from build123d import *

# Parameters (mm, degrees)
F0_W        = 12.9999973349
F0_H        = 13
F0_W_2      = 10
F0_H_2      = 10
F1_DEPTH    = 95
F2_T1_DEPTH = 38
F3_R        = 4
F4_DEPTH    = 2
F5_R        = 7
F5_R_2      = 4
F6_DEPTH    = 2


# Not quite as in the source:
# - a fillet or chamfer that OpenCascade refuses, or shapes differently, is made with other operations: its cross-section is extruded or revolved along the edge and cut away or added


with BuildPart() as f1:
    # F0 (on Right) → F1 (new body)
    with BuildSketch(Plane.YZ):
        with Locations((-12.2499999048, 6.5)):
            Rectangle(F0_W, F0_H)
        with Locations((-12.2499999048, 6.5)):
            Rectangle(F0_W_2, F0_H_2, mode=Mode.SUBTRACT)
    extrude(amount=F1_DEPTH)

    # F2: fillet of radius 5 on 2 edges, made by hand

    # F2_s2 → F2_t1 (cut)
    with BuildSketch(Plane.XY.offset(-12.5)):
        with BuildLine():
            ThreePointArc((90, -5.7500012374), (93.5355339059, -7.2144673315), (95, -10.7500012374))
            Line((95, -10.7500012374), (95, -5.7500012374))
            Line((95, -5.7500012374), (90, -5.7500012374))
        make_face()
        with BuildLine():
            ThreePointArc((90, -18.7499985722), (93.5355339059, -17.2855324782), (95, -13.7499985722))
            Line((95, -13.7499985722), (95, -18.7499985722))
            Line((95, -18.7499985722), (90, -18.7499985722))
        make_face()
    extrude(amount=F2_T1_DEPTH, mode=Mode.SUBTRACT)

    # F3 (on face) → F4 (join)
    with BuildSketch(Plane.XY.offset(13)):
        with Locations((87, -12.2499999048)):
            Circle(F3_R)
    extrude(amount=F4_DEPTH)

    # F5 (on face) → F6 (join)
    with BuildSketch(Plane.XY.offset(15)):
        with Locations((87, -12.2499999048)):
            Circle(F5_R)
        with Locations((87, -12.2499999048)):
            Circle(F5_R_2, mode=Mode.SUBTRACT)
        with Locations((87, -12.2499999048)):
            Circle(F5_R_2)
    extrude(amount=F6_DEPTH)


solid = f1.part
The model under review builds one solid part; all positions refer to its coordinate system, in mm. A direction names the side the tool comes from. Coordinates: 2 decimals unless noted, no trailing zeros. Write each loop counter-clockwise with the first axis right and the second up, starting at its lowest first coordinate (ties: lowest second). Pieces come first, ordered by that corner, then holes. Notation, with made-up numbers: (4.5, 0.25) -> (26.5, 0.25) arc R18 ccw to (26.5, 21.25) -> close; hole circle Ø6 at (-7.75, 76.25). An arc over 180 degrees is marked (long way). Answer in a Markdown table with one row per item.
1. Wall thickness on probe 1 along Z at (x, y) = (8, -9.25); probe 2 along Z at (x, y) = (91.5, -8.75); probe 3 along Y at (x, z) = (18.5, 7.25): over which ranges is each line inside the solid? List them lowest first. Write a range as [from, to].
Answers below:
| item | result |
|---|---|
| probe 1 | z = [0, 1.5], [11.5, 13] |
| probe 2 | z = [0, 1.5], [11.5, 13], [15, 17] |
| probe 3 | y = [-18.75, -17.25], [-7.25, -5.75] |
2. Draft analysis for pull direction Y (two halves, no side actions). For faces 4 (the flat face through (46, -17.25, 6)), 5 (the flat face through (90, -15.3, 15)), 6 (the flat face through (44, -18.75, 6)), state which applies: +Y half, -Y half, draft (parallel to the pull), parting line (faces both ways), or undercut.
Answers below:
| item | result |
|---|---|
| face 4 | undercut |
| face 5 | draft |
| face 6 | -Y half |
3. We need section A-A, the plane z = 2.5. State the section outline as (x, y) points, and give its area (3 significant figures).
Answers below:
| item | result |
|---|---|
| outline | (0, -18.75) -> (90, -18.75) arc R5 ccw to (93.57, -17.25) -> (0, -17.25) -> close; (0, -7.25) -> (93.57, -7.25) arc R5 ccw to (90, -5.75) -> (0, -5.75) -> close |
| area | 277 mm^2 |
4. For faces 1 (the flat face through (47, -12, 1.5)), 2 (the cylindrical face through (80.007, -11.942, 15.986)), 3 (the cylindrical face through (90.695, -13.782, 13.986)), list the 3-axis set-ups (+Z, -Z, +X, -X, +Y, -Y) from which the entire face can be reached by the end or side of a thin tool; tool diameter is ignored.
Answers below:
| item | result |
|---|---|
| face 1 | +X, -X |
| face 2 | +Z |
| face 3 | none |
5. We need section B-B, the plane x = 36.5. State the section outline as (y, z) points.
Answers below:
| item | result |
|---|---|
| outline | (-18.75, 0) -> (-5.75, 0) -> (-5.75, 13) -> (-18.75, 13) -> close; hole (-17.25, 1.5) -> (-7.25, 1.5) -> (-7.25, 11.5) -> (-17.25, 11.5) -> close |
6. We need section D-D, the plane x = 87. State the section outline as (y, z) points.
Answers below:
| item | result |
|---|---|
| outline | (-19.25, 15) -> (-16.25, 15) -> (-16.25, 13) -> (-18.75, 13) -> (-18.75, 0) -> (-5.75, 0) -> (-5.75, 13) -> (-8.25, 13) -> (-8.25, 15) -> (-5.25, 15) -> (-5.25, 17) -> (-19.25, 17) -> close; hole (-17.25, 1.5) -> (-7.25, 1.5) -> (-7.25, 11.5) -> (-17.25, 11.5) -> close |
7. We need section C-C, the plane y = -12.25. State the section outline as (x, z) points, and give its area (3 significant figures).
Answers below:
| item | result |
|---|---|
| outline | (0, 0) -> (95, 0) -> (95, 1.5) -> (0, 1.5) -> close; (0, 11.5) -> (95, 11.5) -> (95, 13) -> (91, 13) -> (91, 15) -> (94, 15) -> (94, 17) -> (80, 17) -> (80, 15) -> (83, 15) -> (83, 13) -> (0, 13) -> close |
| area | 329 mm^2 |
8. Clearance check with flat-ended pins moving along their axes: pin 1 Ø3 at (y, z) = (-15.5, 5.5) entering from -X; pin 2 Ø5 at (x, z) = (35, 4.5) entering from +Y; pin 3 Ø6 at (x, z) = (32, 5.5) entering from -Y; pin 4 Ø1 at (x, y) = (60.5, -17) entering from +Z. State where each tip first meets the part, or that it passes through.
Answers below:
| item | result |
|---|---|
| pin 1 | passes through |
| pin 2 | stops at y = -5.75 |
| pin 3 | stops at y = -18.75 |
| pin 4 | stops at z = 13 |
